Part model, mm, in its own coordinate system. Face numbers are marked on the shaded views. A direction names the side the tool comes from. Round coordinates to 2 decimals unless told otherwise and drop trailing zeros. Write each loop counter-clockwise with the first axis right and the second up, starting at its lowest first coordinate (ties: lowest second). Pieces come first, ordered by that corner, then holes.
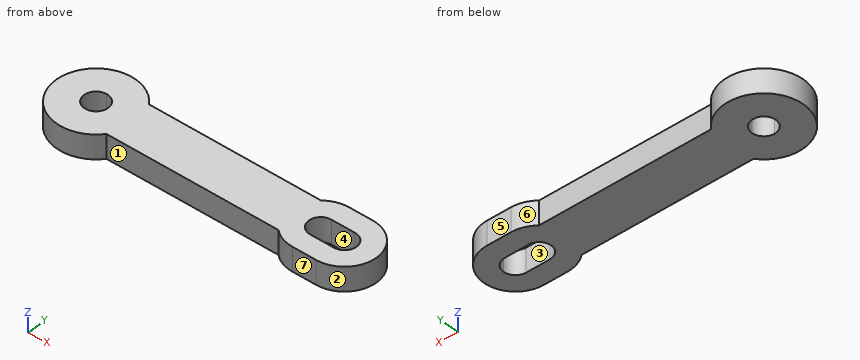
```python
from build123d import *

# Parameters (mm, degrees)
SALIENTE_EXTRUIR2_DEPTH = 3


with BuildPart() as part:
    # Croquis1 → Saliente-Extruir2 (new body)
    # profile 1 of 6: a face of its own
    with BuildSketch(Plane.XY):
        with BuildLine():
            Line((0, -1.5), (0, -3))
            Line((0, -3), (4, -3))
            ThreePointArc((4, -3), (4.74341649, -1.58113883), (5, 0))
            ThreePointArc((5, 0), (4.74341649, 1.58113883), (4, 3))
            Line((4, 3), (0, 3))
            Line((0, 3), (0, 1.5))
            ThreePointArc((0, 1.5), (1.060660172, 1.060660172), (1.5, 0))
            ThreePointArc((1.5, 0), (1.060660172, -1.060660172), (0, -1.5))
        make_face()
    # profile 2 of 6: a face of its own
    with BuildSketch(Plane.XY):
        with BuildLine():
            Line((4, -3), (0, -3))
            Line((0, -3), (0, -1.5))
            ThreePointArc((0, -1.5), (-1.5, 0), (0, 1.5))
            Line((0, 1.5), (0, 3))
            Line((0, 3), (4, 3))
            ThreePointArc((4, 3), (-5, 0), (4, -3))
        make_face()
    # profile 3 of 6: a face of its own
    with BuildSketch(Plane.XY):
        with BuildLine():
            Line((0, -1.5), (0, -3))
            Line((0, -3), (4, -3))
            ThreePointArc((4, -3), (4.74341649, -1.58113883), (5, 0))
            ThreePointArc((5, 0), (4.74341649, 1.58113883), (4, 3))
            Line((4, 3), (0, 3))
            Line((0, 3), (0, 1.5))
            ThreePointArc((0, 1.5), (1.060660172, 1.060660172), (1.5, 0))
            ThreePointArc((1.5, 0), (1.060660172, -1.060660172), (0, -1.5))
        make_face()
    # profile 4 of 6: a face of its own
    with BuildSketch(Plane.XY):
        with BuildLine():
            Line((4, -3), (0, -3))
            Line((0, -3), (0, -1.5))
            ThreePointArc((0, -1.5), (-1.5, 0), (0, 1.5))
            Line((0, 1.5), (0, 3))
            Line((0, 3), (4, 3))
            ThreePointArc((4, 3), (-5, 0), (4, -3))
        make_face()
    # profile 5 of 6: a face of its own
    with BuildSketch(Plane.XY):
        with BuildLine():
            ThreePointArc((5, 0), (4.74341649, -1.58113883), (4, -3))
            Line((4, -3), (25.754248689, -3))
            ThreePointArc((25.754248689, -3), (24.4, 0), (25.754248689, 3))
            Line((25.754248689, 3), (4, 3))
            ThreePointArc((4, 3), (4.74341649, 1.58113883), (5, 0))
        make_face()
    # profile 6 of 6: a face of its own
    with BuildSketch(Plane.XY):
        with BuildLine():
            ThreePointArc((25.754248689, 3), (24.4, 0), (25.754248689, -3))
            ThreePointArc((25.754248689, -3), (26.985786438, -3.741657387), (28.4, -4))
            Line((28.4, -4), (31.4, -4))
            ThreePointArc((31.4, -4), (35.4, 0), (31.4, 4))
            Line((31.4, 4), (28.4, 4))
            ThreePointArc((28.4, 4), (26.985786438, 3.741657387), (25.754248689, 3))
        make_face()
        with BuildLine():
            Line((31.4, -1.5), (28.4, -1.5))
            ThreePointArc((28.4, -1.5), (26.9, 0), (28.4, 1.5))
            Line((28.4, 1.5), (31.4, 1.5))
            ThreePointArc((31.4, 1.5), (32.460660172, 1.060660172), (32.9, 0))
            ThreePointArc((32.9, 0), (32.460660172, -1.060660172), (31.4, -1.5))
        make_face(mode=Mode.SUBTRACT)
    extrude(amount=SALIENTE_EXTRUIR2_DEPTH)


solid = part.part
```
Q1. Cut at B-B on z = 2.1. Write the cut outline in (x, y), plus the area to 3 significant figures.
Values follow:
outline: (4, -3) - (25.75, -3) arc R4 ccw to (28.4, -4) - (31.4, -4) arc R4 ccw to (31.4, 4) - (28.4, 4) arc R4 ccw to (25.75, 3) - (4, 3) arc R5 ccw (long way) to start; hole circle Ø3 at (0, 0); hole (28.4, -1.5) - (31.4, -1.5) arc R1.5 ccw to (31.4, 1.5) - (28.4, 1.5) arc R1.5 ccw to start
area: 250 mm2
Q2. Drop flat-ended pins along their axis: pin 1 (0.9 mm diameter, centred on x = 30, z = 1.5, fed in from -Y); pin 2 (0.9 mm diameter, centred on x = 29.5, z = 1, fed in from +Y); pin 3 (1 mm diameter, centred on x = 5.5, y = 4, fed in from +Z). Give the stop position or say it passes through.
Values follow:
pin 1: stops at y = -4
pin 2: stops at y = 4
pin 3: passes through
Q3. Cut at C-C on y = -3.5. Write the cut outline in (x, z), plus the area to 3 significant figures.
Values follow:
outline: (-3.57, 0) - (3.57, 0) - (3.57, 3) - (-3.57, 3) - close; (26.46, 0) - (33.34, 0) - (33.34, 3) - (26.46, 3) - close
area: 42.0 mm2
Q4. Which spindle directions (+Z, -Z, +X, -X, +Y, -Y) get a long thin tool onto all of the face, cutting with end or side? Do the marked faces 4, 5, 6 and 7. Say none if no direction does.
Values follow:
face 4: +Z, -Z
face 5: +Z, -Z, +X, +Y
face 6: +Z, -Z, +Y
face 7: +Z, -Z, +X, -Y
Q5. Cut at A-A on y = 0.5. Write the cut outline in (x, z), plus the area to 3 significant figures.
Values follow:
outline: (-4.97, 0) - (-1.41, 0) - (-1.41, 3) - (-4.97, 3) - close; (1.41, 0) - (26.99, 0) - (26.99, 3) - (1.41, 3) - close; (32.81, 0) - (35.37, 0) - (35.37, 3) - (32.81, 3) - close
area: 95.1 mm2
Q6. Cut at D-D on x = 12. Write the cut outline in (y, z), plus the area to 3 significant figures.
Values follow:
outline: (-3, 0) - (3, 0) - (3, 3) - (-3, 3) - close
area: 18.0 mm2
Q7. Mould opens along Y. For the marked faces 1, 2 and 3 say: +Y half, -Y half, draft (parallel to the pull), parting line (faces both ways), or undercut.
Values follow:
face 1: -Y half
face 2: parting line
face 3: undercut
Q8. Wall check: L1, parallel to Y at x = 25.5, z = 2.45; L2, parallel to Y at x = 28, z = 0.7; L3, parallel to X at y = -3.5, z = 1.75. Give the ranges that are in metal, low to high.
Values follow:
L1: y = -3 to 3
L2: y = -3.98 to -1.45, 1.45 to 3.98
L3: x = -3.57 to 3.57, 26.46 to 33.34
